Can you work these out from the model? Positions are in its coordinate system, mm. A direction names the side the tool comes from. Round coordinates to 2 decimals unless told otherwise and drop trailing zeros. Write each loop counter-clockwise with the first axis right and the second up, starting at its lowest first coordinate (ties: lowest second). Pieces come first, ordered by that corner, then holes. Notation, with made-up numbers: (-13.75, 85.25) -> (-6.75, 85.25) arc R32 ccw to (-6.75, 122.25) -> close; hole circle Ø11 at (42.5, 75). An arc over 180 degrees is marked (long way). Write item = value, one per line. Start each with the question number.
1) Imagine slicing it at C-C, the plane x = -34. Please give me the cut outline in (y, z), then the cut area to 3 significant figures.
2) Imagine slicing it at A-A, the plane x = -17. Please give me the cut outline in (y, z).
3) I'm going to push flat-ended pins straight in: pin 1 (9 mm diameter, centred on x = -17, y = -25, fed in from +Z); pin 2 (13 mm diameter, centred on x = -131.82, y = 7.63, fed in from -Z); pin 3 (8 mm diameter, centred on x = -63, z = -2.5, fed in from +Y); pin 4 (1 mm diameter, centred on y = -5, z = 4.5, fed in from -X). Where does each tip first touch, or does it pass through?
4) Thinking about a two-plate mould opening in Y: for faces 4 (the face through (-46, 0, 0)), 5 (the face through (-25, -7, -4)), 6 (the face through (-124.22, -25.59, 3.94)), 7 (the face through (-70, -25, -4)), which applies, +Y half, -Y half, draft (parallel to the pull), parting line (faces both ways), or undercut?
5) If I drill on line 1 (Y direction, x = -17, z = 4.25); line 2 (X direction, y = -17, z = -2.5); line 3 (Z direction, x = -21, y = -30), over which ranges is the centre line in solid material (lowest first)?
6) Imagine slicing it at D-D, the plane z = -1.5. Please give me the cut outline in (x, y).
7) Imagine slicing it at B-B, the plane z = 5. Please give me the cut outline in (x, y), then the cut area to 3 significant figures.
8) For faces 1 (the face through (-25, -25, 0)), 2 (the face through (0, -25, 2)), 3 (the face through (-110, -12, 0)), which set-ups out of +Z, -Z, +X, -X, +Y, -Y let a thin tool reach every point of the face, with its end or its side?
Autodesk Inventor part; units mm, degrees
ref_plane "YZ Plane" through (0, 0, 0) normal (1, 0, 0) x (0, 1, 0)
ref_plane "XZ Plane" through (0, 0, 0) normal (0, 1, 0) x (-1, 0, 0)
ref_plane "XY Plane" through (0, 0, 0) normal (0, 0, 1) x (1, 0, 0)
sketch "Sketch1" plane through (0, 0, 0) normal (0, 0, 1) x (1, 0, 0)
  line L0 (0, 0) -> (-100, 0)
  line L1 (-100, 0) -> (-100, -50)
  line L2 (-100, -50) -> (0, -50)
  line L3 (0, -50) -> (0, 0)
  line L4 (0, 0) -> (-70, 0)
  line L5 (-70, 0) -> (-70, -50)
  line L6 (-70, -50) -> (0, -50)
  line L7 (0, -50) -> (0, 0)
  line L8 (0, -7) -> (-50, -7)
  line L9 (-50, -7) -> (-50, -43)
  line L10 (-50, -43) -> (0, -43)
  line L11 (0, -43) -> (0, -7)
  line L12 (-100, -24.1908) -> (-131.8198, 7.629)
  line L13 (-100, -24.1908) -> (-55, -24.1908) construction
  circle A0 centre (-131.8198, 7.629) radius 5
  circle A1 centre (-100, -24.1908) radius 5
  circle A2 centre (-17, -25) radius 5
  circle A3 centre (-131.8198, 7.629) radius 18
  line L14 (-100, 0) -> (-118.6863, 19.938)
  line L15 (-100, -50) -> (-144.5979, -5.0486)
  point P0 (0, -43)
  dimension "d0" = 100
  dimension "d1" = 50
  dimension "d2" = 36
  dimension "d3" = 50
  dimension "d4" = 7
  dimension "d5" = 45
  dimension "d6" = 135
  dimension "d7" = 10
  dimension "d8" = 36
  dimension "d9" = 17
  dimension "d10" = 25
  dimension "d11" = 70
  dimension "d13" = 133.144
extrude "Extrusion1" add sketch "Sketch1" along normal blind 8 contours L3 L8 L9 L10 L2 L5 L0 | L5 L2 L1 A1 L0 | L3 L10 L9 L8 | L1 A1 L12 A3 L14 | A3 | L15 A3 L12 A1 L1
extrude "Extrusion2" add sketch "Sketch1" against normal blind 8 contours L3 L8 L9 L10 L2 L5 L0
fillet "Fillet1" radius 15 2 edges at (-100, 0, 4) (-100, -50, 4)
properties part number "handlesupport" material "Steel, Mild"
Reported:
q1.outline = (-50, -8) -> (-43, -8) -> (-43, 0) -> (-7, 0) -> (-7, -8) -> (0, -8) -> (0, 8) -> (-50, 8) -> close
q1.area = 512 mm²
q2.outline = (-50, -8) -> (-43, -8) -> (-43, 0) -> (-30, 0) -> (-30, 8) -> (-50, 8) -> close; (-20, 0) -> (-7, 0) -> (-7, -8) -> (0, -8) -> (0, 8) -> (-20, 8) -> close
q3.pin_1 = through
q3.pin_2 = 0
q3.pin_3 = 0
q3.pin_4 = -145.12
q4.face_4 = +Y half
q4.face_5 = undercut
q4.face_6 = -Y half
q4.face_7 = draft
q5.line_1 = -50 to -30, -20 to 0
q5.line_2 = -70 to -50
q5.line_3 = 0 to 8
q6.outline = (-70, -50) -> (0, -50) -> (0, -43) -> (-50, -43) -> (-50, -7) -> (0, -7) -> (0, 0) -> (-70, 0) -> close
q7.outline = (-144.6, -5.05) -> (-104.4, -45.56) arc R15 ccw to (-93.75, -50) -> (0, -50) -> (0, 0) -> (-93.5, 0) arc R15 cw to (-104.44, 4.74) -> (-118.69, 19.94) arc R18 ccw (long way) to start; hole circle Ø10 at (-131.82, 7.63); hole circle Ø10 at (-100, -24.19); hole circle Ø10 at (-17, -25)
q7.area = 6,890 mm²
q8.face_1 = -Z, +X
q8.face_2 = +Z, -Z, +X, +Y, -Y
q8.face_3 = -Z, -X, +Y, -Y
